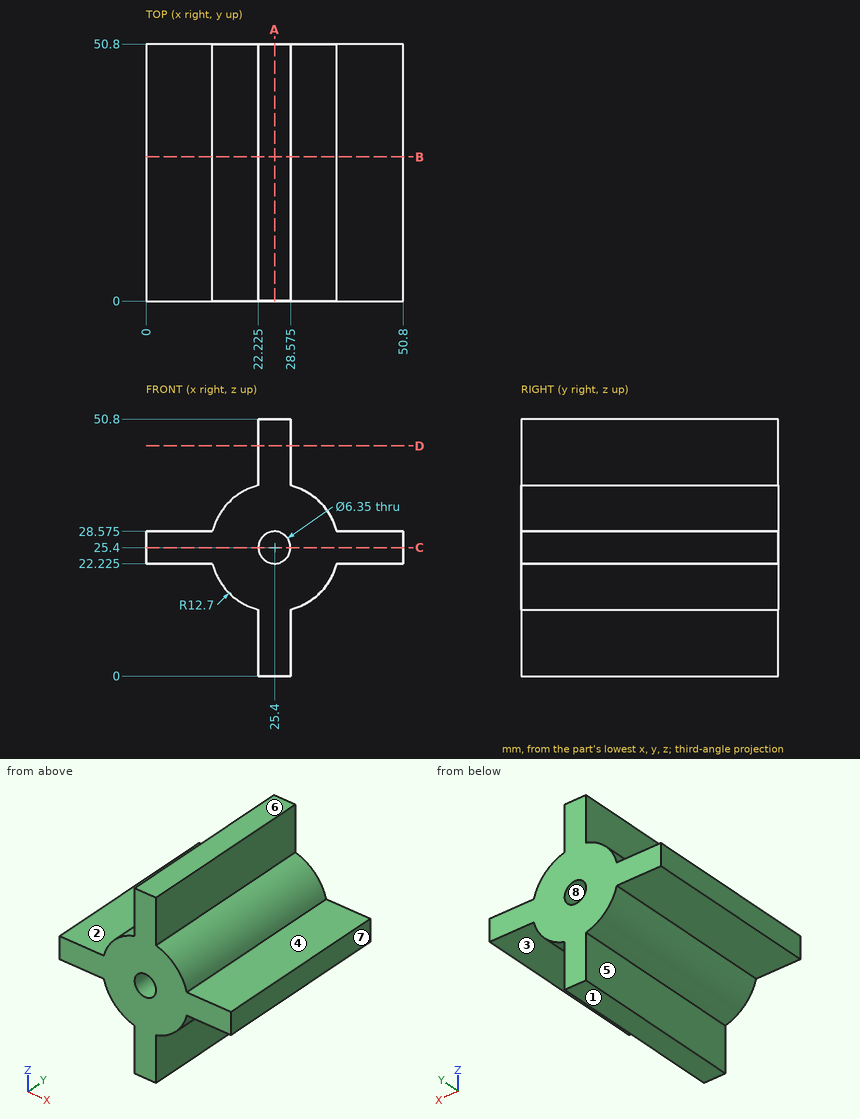
Part print with two shaded views. Sizes in mm from the minimum x, y, z corner. A direction names the side the tool comes from. Give positions to 0.01 mm unless a question says otherwise; leave off trailing zeros. Loops run counter-clockwise (first coordinate to the right, second up) from the corner with the lowest first, then second, coordinate; pieces in that order, holes last. Notation, with made-up numbers: (71, 51) - (117, 51) arc R24 ccw to (117, 66) - close; hole circle Ø7 at (14, 44.25). An arc over 180 degrees is marked (long way). Put each result on its own line as item: value.
Q1. Probe line 1 along Z through (x, y) = (25.4, 30) (3 decimals); line 2 along Z through (x, y) = (43.5, 37) (3 decimals). List the from-to ranges inside material, lowest first.
Filled in:
line 1: z = 0 to 22.225, 28.575 to 50.8
line 2: z = 22.225 to 28.575
Q2. Slice it at D-D (z = 45.5). Give the cut face in (x, y) (3 decimals).
Filled in:
outline: (22.225, 0) - (28.575, 0) - (28.575, 50.8) - (22.225, 50.8) - close
Q3. Flat gauge pins, fed straight in: pin 1 (4 mm diameter, centred on x = 18, y = 24, fed in from -Z); pin 2 (10.5 mm diameter, centred on y = 14, z = 43.5, fed in from +X) (3 decimals); pin 3 (4 mm diameter, centred on y = 11.5, z = 44.5, fed in from -X) (3 decimals); pin 4 (5 mm diameter, centred on x = 25.4, z = 25.4, fed in from +Y). Where does each tip first touch, or does it go through?
Filled in:
pin 1: stops at z = 13.91
pin 2: stops at x = 28.575
pin 3: stops at x = 22.225
pin 4: passes through
Q4. Mould opens along X. For the marked faces 6, 7 and 8 say: pulls with the +X half, pulls with the -X half, needs draft (parallel to the pull), parting line crosses it, or undercut.
Filled in:
face 6: needs draft
face 7: pulls with the +X half
face 8: undercut
Q5. Slice it at C-C (z = 25.4). Give the cut face in (x, y) (3 decimals), plus the area to 3 significant figures.
Filled in:
outline: (0, 0) - (22.225, 0) - (22.225, 50.8) - (0, 50.8) - close; (28.575, 0) - (50.8, 0) - (50.8, 50.8) - (28.575, 50.8) - close
area: 2,260 mm²
Q6. Tool access for the marked faces 1, 2, 3, 4 and 5: list every direction of +Z, -Z, +X, -X, +Y, -Y with a clear straight run to the whole face (end or side of a thin tool).
Filled in:
face 1: -Z, +X, -X, +Y, -Y
face 2: +Z, -X, +Y, -Y
face 3: -Z, +X, +Y, -Y
face 4: +Z, +X, +Y, -Y
face 5: -Z, -X, +Y, -Y
Q7. Slice it at A-A (x = 25.4). Give the cut face in (y, z) (3 decimals), plus the area to 3 significant figures.
Filled in:
outline: (0, 0) - (50.8, 0) - (50.8, 22.225) - (0, 22.225) - close; (0, 28.575) - (50.8, 28.575) - (50.8, 50.8) - (0, 50.8) - close
area: 2,260 mm²
Q8. Slice it at B-B (y = 28.5). Give the cut face in (x, z) (3 decimals).
Filled in:
outline: (0, 22.225) - (13.103, 22.225) arc R12.7 ccw to (22.225, 13.103) - (22.225, 0) - (28.575, 0) - (28.575, 13.103) arc R12.7 ccw to (37.697, 22.225) - (50.8, 22.225) - (50.8, 28.575) - (37.697, 28.575) arc R12.7 ccw to (28.575, 37.697) - (28.575, 50.8) - (22.225, 50.8) - (22.225, 37.697) arc R12.7 ccw to (13.103, 28.575) - (0, 28.575) - close; hole circle Ø6.35 at (25.4, 25.4)
